Geometry: final body of the model. Coordinates: model frame, mm. A direction names the side the tool comes from. Give positions to 0.01 mm unless a question says otherwise; leave off trailing zeros. Write each loop counter-clockwise with the first axis right and the second up, starting at its lowest first coordinate (ties: lowest second). Pieces come first, ordered by that corner, then holes. Notation, with made-up numbers: M 34,18 L 42,18 A12 ccw 42,40 Z; hole C 46,62.25 d11. An arc over 180 degrees is marked long. Use a Markdown table: item, result. Add a question column.
(1) Material intervals for L1, parallel to Z at x = 30, y = 4.55; L2, parallel to X at y = 3.05, z = 0; L3, parallel to Z at x = 27.5, y = 3.3, sorted ascending.
(2) Cut plane D-D (z = -11.5). Output: boundary loops of the cut face in (x, y).
(3) Pin query (flat end, axial travel): pin 1 Ø2 at (x, y) = (-58, 1.5) entering from +Z; pin 2 Ø2.5 at (x, z) = (0, 0) entering from -Y; pin 3 Ø1 at (x, y) = (47, 4) entering from +Z; pin 4 Ø2 at (x, y) = (67, 4) entering from -Z. Return the tip coordinate at first contact, or that it passes through.
(4) Cut plane B-B (z = -73). Output: boundary loops of the cut face in (x, y), plus the area to 3 significant figures.
(5) Cut plane A-A (y = 3.5). State how many separate pieces and enclosed holes the cut face has, plus the area to 3 significant figures.
(6) Reachability of faces 1 (the flat face through (-1.3, 0, -1.3)), 2 (the cylindrical face through (5.06, 2.46, -82.21)) from +Z, -Z, +X, -X, +Y, -Y: full face, straight path, thin tool, end or side. Return the list, or none.
(7) Draft query along X for faces 3 (the flat face through (1.3, 5, -1.3)), 4 (the cylindrical face through (-55.504, 2.535, 24.294)), 5 (the cylindrical face through (-90.3, 2.46, -20.05)). Return one class per face: released by +X, released by -X, zero draft, split by the parting line, or undercut.
(8) Cut plane C-C (x = 31.5). Output: boundary loops of the cut face in (y, z), plus the area to 3 significant figures.
```python
from build123d import *

# Parameters (mm, degrees)
SKETCH_1_R             = 92.5
SKETCH_1_R_2           = 1.5
EXTRUDE_1_DEPTH        = 5
CUT_EXTRUDE_1_DEPTH    = 30
FILLET_3_R             = 10
SKETCH_1_3_R           = 1.5
EXTRUDE_2_DEPTH        = 5
SKETCH_1_5_OUTSIDE_W   = 239.336
SKETCH_1_5_OUTSIDE_H   = 239.336
SKETCH_1_5_OUTSIDE_R   = 92.5
SKETCH_1_5_OUTSIDE_R_2 = 1.5
CUT_EXTRUDE_2_DEPTH    = 5


with BuildPart() as part:
    # 草图1 → 凸台-拉伸1 (new body)
    with BuildSketch(Plane(origin=(0, 0, 0), x_dir=(1, 0, 0), z_dir=(0, 1, 0))):
        with Locations(Location((0, 0, 0), (0, 0, 270))):
            Circle(SKETCH_1_R)
        with Locations(Location((0, 0, 0), (0, 0, 270))):
            Circle(SKETCH_1_R_2, mode=Mode.SUBTRACT)
        with Locations(Location((0, 7, 0), (0, 0, 270))):
            Circle(SKETCH_1_R_2, mode=Mode.SUBTRACT)
        with Locations(Location((7, 0, 0), (0, 0, 270))):
            Circle(SKETCH_1_R_2, mode=Mode.SUBTRACT)
        with Locations(Location((0, -7, 0), (0, 0, 270))):
            Circle(SKETCH_1_R_2, mode=Mode.SUBTRACT)
        with Locations(Location((-7, 0, 0), (0, 0, 270))):
            Circle(SKETCH_1_R_2, mode=Mode.SUBTRACT)
    extrude(amount=EXTRUDE_1_DEPTH)

    # 草图2 → 切除-拉伸1 (cut)
    with BuildSketch(Plane(origin=(0, 5, 0), x_dir=(1, 0, 0), z_dir=(0, 1, 0))):
        with BuildLine():
            Line((2.591280941, 86.258429639), (-2.591280941, 66.941570361))
            ThreePointArc((-2.591280941, 66.941570361), (35.5302713, 22.943474897), (8.881266501, -28.814767857))
            Line((8.881266501, -28.814767857), (18.480344966, -46.360641806))
            ThreePointArc((18.480344966, -46.360641806), (55.388254532, 25.322655836), (2.591280941, 86.258429639))
        make_face()
        with BuildLine():
            Line((-8.881266501, 28.814767857), (-18.480344966, 46.360641806))
            ThreePointArc((-18.480344966, 46.360641806), (-55.388254532, -25.322655836), (-2.591280941, -86.258429639))
            Line((-2.591280941, -86.258429639), (2.591280941, -66.941570361))
            ThreePointArc((2.591280941, -66.941570361), (-35.5302713, -22.943474897), (-8.881266501, 28.814767857))
        make_face()
    extrude(amount=-CUT_EXTRUDE_1_DEPTH, mode=Mode.SUBTRACT)

    # 圆角3
    fillet_3_edges = [part.edges().sort_by_distance(p)[0] for p in [
        (-18.480344966, 2.5, -46.360641806),
        (-8.881266501, 2.5, -28.814767857),
        (-2.591280941, 2.5, 86.258429639),
        (2.591280941, 2.5, 66.941570361),
        (18.480344966, 2.5, 46.360641806),
        (8.881266501, 2.5, 28.814767857),
        (-2.591280941, 2.5, -66.941570361),
        (2.591280941, 2.5, -86.258429639),
    ]]
    fillet(fillet_3_edges, radius=FILLET_3_R - 0.0001)  # a hair under: the kernel refuses the full size

    # 草图1<3> → 凸台-拉伸2 (add)
    with BuildSketch(Plane(origin=(0, 0, 0), x_dir=(1, 0, 0), z_dir=(0, 1, 0))):
        Circle(SKETCH_1_3_R)
    extrude(amount=EXTRUDE_2_DEPTH)

    # 草图1<5> outside → 切除-拉伸2 (cut)
    # profile 1 of 6: a face of its own
    with BuildSketch(Plane(origin=(0, 0, 0), x_dir=(1, 0, 0), z_dir=(0, 1, 0))):
        Rectangle(SKETCH_1_5_OUTSIDE_W, SKETCH_1_5_OUTSIDE_H)
        with Locations(Location((0, 0, 0), (0, 0, 270))):
            Circle(SKETCH_1_5_OUTSIDE_R, mode=Mode.SUBTRACT)
    # profile 2 of 6: a face of its own
    with BuildSketch(Plane(origin=(0, 0, 0), x_dir=(1, 0, 0), z_dir=(0, 1, 0))):
        with Locations(Location((0, 0, 0), (0, 0, 270))):
            Circle(SKETCH_1_5_OUTSIDE_R_2)
    # profile 3 of 6: a face of its own
    with BuildSketch(Plane(origin=(0, 0, 0), x_dir=(1, 0, 0), z_dir=(0, 1, 0))):
        with Locations(Location((0, 7, 0), (0, 0, 270))):
            Circle(SKETCH_1_5_OUTSIDE_R_2)
    # profile 4 of 6: a face of its own
    with BuildSketch(Plane(origin=(0, 0, 0), x_dir=(1, 0, 0), z_dir=(0, 1, 0))):
        with Locations(Location((7, 0, 0), (0, 0, 270))):
            Circle(SKETCH_1_5_OUTSIDE_R_2)
    # profile 5 of 6: a face of its own
    with BuildSketch(Plane(origin=(0, 0, 0), x_dir=(1, 0, 0), z_dir=(0, 1, 0))):
        with Locations(Location((0, -7, 0), (0, 0, 270))):
            Circle(SKETCH_1_5_OUTSIDE_R_2)
    # profile 6 of 6: a face of its own
    with BuildSketch(Plane(origin=(0, 0, 0), x_dir=(1, 0, 0), z_dir=(0, 1, 0))):
        with Locations(Location((-7, 0, 0), (0, 0, 270))):
            Circle(SKETCH_1_5_OUTSIDE_R_2)
    extrude(amount=CUT_EXTRUDE_2_DEPTH, mode=Mode.SUBTRACT)


solid = part.part
```
Answer list:
| question | item | result |
|---|---|---|
| 1 | L1 | -87.5 to -72.05, -40.81 to 7.28, 38.52 to 87.5 |
| 1 | L2 | -92.5 to -53.92, -33.12 to -8.5, -5.5 to -1.5, 1.5 to 5.5, 8.5 to 33.12, 53.92 to 92.5 |
| 1 | L3 | -88.32 to -74.04, -45.09 to 11.56, 40.47 to 88.32 |
| 2 | outline | M -91.78,0 L -50.12,0 L -50.12,5 L -91.78,5 Z; M -27.54,0 L 35.63,0 L 35.63,5 L -27.54,5 Z; M 55.71,0 L 91.78,0 L 91.78,5 L 55.71,5 Z |
| 3 | pin 1 | z = 72.85 |
| 3 | pin 2 | through |
| 3 | pin 3 | z = 79.96 |
| 3 | pin 4 | z = -64.81 |
| 4 | outline | M -56.81,0 L -0.55,0 L -0.55,5 L -56.81,5 Z; M 28.83,0 L 56.81,0 L 56.81,5 L 28.83,5 Z |
| 4 | area | 421 mm² |
| 5 | separate pieces | 1 |
| 5 | enclosed holes | 7 |
| 5 | area | 21,100 mm² |
| 6 | face 1 | +Z, -Z, +X, -X, -Y |
| 6 | face 2 | +Y, -Y |
| 7 | face 3 | zero draft |
| 7 | face 4 | undercut |
| 7 | face 5 | split by the parting line |
| 8 | outline | M 0,-86.97 L 5,-86.97 L 5,-70.76 L 0,-70.76 Z; M 0,-37.69 L 5,-37.69 L 5,4.16 L 0,4.16 Z; M 0,37.24 L 5,37.24 L 5,86.97 L 0,86.97 Z |
| 8 | area | 539 mm² |
